Design review of the part built by this model. Coordinates are the model's own, in mm. Give positions to 0.01 mm unless a question says otherwise; leave off trailing zeros. Loops run counter-clockwise (first coordinate to the right, second up) from the corner with the lowest first, then second, coordinate; pieces in that order, holes last. Notation, with made-up numbers: M 46.5,44 L 105.5,44 A22 ccw 105.5,59 Z; hole C 70.5,-1 d9. An arc over 180 degrees is marked long. Answer as CSV lines item,"result".
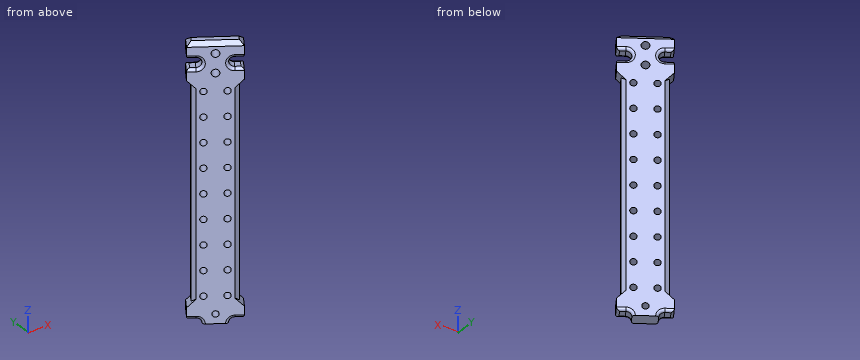
```python
from build123d import *

# Parameters (mm, degrees)
BOSS_EXTRU_1_OUTLINE_R   = 2.75
BOSS_EXTRU_1_OUTLINE_R_2 = 2.3
BOSS_EXTRU_1_DEPTH       = 10
ESQUISSE2_R              = 2.3
ENL_V_MAT_EXTRU_1_DEPTH  = 192.889965503
CONG_1_R                 = 2
CHANFREIN1_SIZE          = 3


# Read off the part's stored shape, not the designer's step: Boss.-Extru.1
with BuildPart() as part:
    # Boss.-Extru.1 outline → Boss.-Extru.1 (new body)
    with BuildSketch(Plane(origin=(0.807648755, 1.292238009, 0), x_dir=(0.8479983040028684, -0.5299989400067315, 0), z_dir=(0.5299989400067315, 0.8479983040028684, 0))):
        with BuildLine():
            Line((-3.319738136, 183.05), (-9.244866887, 183.05))
            ThreePointArc((-9.244866887, 183.05), (-11.896517316, 184.148349571), (-12.994866887, 186.8))
            Line((-12.994866887, 186.8), (-29.644053825, 186.8))
            ThreePointArc((-29.644053825, 186.8), (-30.742403396, 184.148349571), (-33.394053825, 183.05))
            Line((-33.394053825, 183.05), (-39.319182576, 183.05))
            Line((-39.319182576, 183.05), (-39.319182576, 174.8))
            Line((-39.319182576, 174.8), (-36.319182576, 171.8))
            Line((-36.319182576, 171.8), (-36.319182576, 15))
            Line((-36.319182576, 15), (-39.319182576, 12))
            Line((-39.319182576, 12), (-39.319182576, 3.75))
            Line((-39.319182576, 3.75), (-33.394053825, 3.75))
            ThreePointArc((-33.394053825, 3.75), (-29.644053825, 0), (-33.394053825, -3.75))
            Line((-33.394053825, -3.75), (-39.319182576, -3.75))
            Line((-39.319182576, -3.75), (-39.319182576, -12))
            Line((-39.319182576, -12), (-36.319182576, -15))
            Line((-36.319182576, -15), (-6.319738136, -15))
            Line((-6.319738136, -15), (-3.319738136, -12))
            Line((-3.319738136, -12), (-3.319738136, -3.75))
            Line((-3.319738136, -3.75), (-9.244866887, -3.75))
            ThreePointArc((-9.244866887, -3.75), (-12.994866887, 0), (-9.244866887, 3.75))
            Line((-9.244866887, 3.75), (-3.319738136, 3.75))
            Line((-3.319738136, 3.75), (-3.319738136, 12))
            Line((-3.319738136, 12), (-6.319738136, 15))
            Line((-6.319738136, 15), (-6.319738136, 171.8))
            Line((-6.319738136, 171.8), (-3.319738136, 174.8))
            Line((-3.319738136, 174.8), (-3.319738136, 183.05))
        make_face()
        with Locations((-21.319460356, -7)):
            Circle(BOSS_EXTRU_1_OUTLINE_R, mode=Mode.SUBTRACT)
        with Locations((-21.319460356, 7)):
            Circle(BOSS_EXTRU_1_OUTLINE_R, mode=Mode.SUBTRACT)
        with Locations((-21.319460356, 179.8)):
            Circle(BOSS_EXTRU_1_OUTLINE_R_2, mode=Mode.SUBTRACT)
    extrude(amount=BOSS_EXTRU_1_DEPTH)

    # Esquisse2 → Enlèv. mat.-Extru.1 (cut, through all)
    with BuildSketch(Plane(origin=(6.107638155, 9.772221049, 0), x_dir=(0.8479983040028684, -0.5299989400067316, 0), z_dir=(0.5299989400067316, 0.8479983040028684, 0))):
        with Locations(Location((-28.819321466, 148.45, 0), (0, 0, 180))):
            Circle(ESQUISSE2_R)
        with Locations(Location((-13.819599246, 148.45, 0), (0, 0, 180))):
            Circle(ESQUISSE2_R)
        with Locations(Location((-28.819321466, 130.1, 0), (0, 0, 180))):
            Circle(ESQUISSE2_R)
        with Locations(Location((-13.819599246, 130.1, 0), (0, 0, 180))):
            Circle(ESQUISSE2_R)
        with Locations(Location((-28.819321466, 111.75, 0), (0, 0, 180))):
            Circle(ESQUISSE2_R)
        with Locations(Location((-13.819599246, 111.75, 0), (0, 0, 180))):
            Circle(ESQUISSE2_R)
        with Locations(Location((-28.819321466, 93.4, 0), (0, 0, 180))):
            Circle(ESQUISSE2_R)
        with Locations(Location((-13.819599246, 93.4, 0), (0, 0, 180))):
            Circle(ESQUISSE2_R)
        with Locations(Location((-28.819321466, 75.05, 0), (0, 0, 180))):
            Circle(ESQUISSE2_R)
        with Locations(Location((-13.819599246, 75.05, 0), (0, 0, 180))):
            Circle(ESQUISSE2_R)
        with Locations(Location((-13.819599246, 56.7, 0), (0, 0, 180))):
            Circle(ESQUISSE2_R)
        with Locations(Location((-13.819599246, 38.35, 0), (0, 0, 180))):
            Circle(ESQUISSE2_R)
        with Locations(Location((-13.819599246, 20, 0), (0, 0, 180))):
            Circle(ESQUISSE2_R)
        with Locations(Location((-28.819321466, 38.35, 0), (0, 0, 180))):
            Circle(ESQUISSE2_R)
        with Locations(Location((-28.819321466, 20, 0), (0, 0, 180))):
            Circle(ESQUISSE2_R)
        with Locations(Location((-28.819321466, 56.7, 0), (0, 0, 180))):
            Circle(ESQUISSE2_R)
        with Locations(Location((-28.819321466, 166.8, 0), (0, 0, 180))):
            Circle(ESQUISSE2_R)
        with Locations(Location((-13.819599246, 166.8, 0), (0, 0, 180))):
            Circle(ESQUISSE2_R)
    extrude(amount=-ENL_V_MAT_EXTRU_1_DEPTH, mode=Mode.SUBTRACT)

    # Congé1
    cong_1_edges = [part.edges().sort_by_distance(p)[0] for p in [
        (0.78025628, 13.10183472, 3.75),
        (-4.911986926, 16.659486724, 0),
        (0.78025628, 13.10183472, -3.75),
        (-3.980588352, 16.077362616, -184.148349571),
        (0.78025628, 13.10183472, -183.05),
        (-19.961867785, 26.065662262, -184.148349571),
        (-24.722712418, 29.041190157, -183.05),
        (-4.51973312, 4.62185168, -183.05),
        (-4.51973312, 4.62185168, -3.75),
        (-10.211976326, 8.179503684, 0),
        (-4.51973312, 4.62185168, 3.75),
        (-30.022701818, 20.561207117, 3.75),
        (-24.330458612, 17.003555113, 0),
        (-30.022701818, 20.561207117, -3.75),
        (-30.022701818, 20.561207117, -183.05),
        (-25.261857185, 17.585679222, -184.148349571),
        (-9.280577752, 7.597379576, -184.148349571),
        (0.642511146, 7.291687222, -183.05),
        (0.642511146, 7.291687222, -3.75),
        (0.642511146, 7.291687222, 3.75),
        (-29.884956684, 26.371354616, 3.75),
        (-29.884956684, 26.371354616, -3.75),
        (-29.884956684, 26.371354616, -183.05),
        (-24.722712418, 29.041190157, -3.75),
        (-19.030469212, 25.483538153, 0),
        (-24.722712418, 29.041190157, 3.75),
    ]]
    fillet(cong_1_edges, radius=CONG_1_R)

    # Chanfrein1
    chanfrein1_edges = [part.edges().sort_by_distance(p)[0] for p in [
        (0.748510934, 13.121675562, -93.4),
        (-4.551478466, 4.641692522, -93.4),
        (-17.271217469, 12.591529399, 15),
        (-29.990956472, 20.541366276, -93.4),
        (-24.690967072, 29.021349316, -93.4),
        (-11.971228069, 21.071512439, 15),
    ]]
    chamfer(chanfrein1_edges, length=CHANFREIN1_SIZE)


solid = part.part
```
1. To check wall thickness, follow L1, parallel to Z at x = -14, y = 21.5; L2, parallel to X at y = 9.75, z = -45; L3, parallel to Z at x = -17, y = 21.5. State the ranges of each line that lie inside material, in increasing order. Write a range as [from, to].
Answer block:
L1,"[-186.8, -181.02], [-178.58, -8.94], [-5.06, 5.06], [8.94, 12.71]"
L2,"[-12.72, -1.36]"
L3,"[-186.8, 14.3]"
2. For P1, Ø12, axis at y = 10.5, z = -144.5, coming from the -X side; P2, Ø2, axis at y = 18, z = -100.5, coming from the -X side; P3, Ø6, axis at y = 6, z = -79.5, coming from the -X side, all flat-tipped, find the tip position at first contact; note any pin that passes through.
Answer block:
P1,"x = -23.52"
P2,"x = -27.46"
P3,"x = -11.52"
3. We need section A-A, the plane z = -126. Write out the cut boundary in (x, y), plus the area to 3 significant figures.
Answer block:
outline,"M -28.4,23.09 L -27.45,18.95 L -7.1,6.23 L -2.96,7.19 L -0.84,10.58 L -1.8,14.71 L -22.15,27.43 L -26.28,26.48 Z"
area,"282 mm²"
